Part model, mm, in its own coordinate system. Round coordinates to 2 decimals unless told otherwise and drop trailing zeros. Loops run counter-clockwise (first coordinate to the right, second up) from the corner with the lowest first, then second, coordinate; pieces in that order, holes last.
from build123d import *

# Parameters (mm, degrees)
SKETCH1_W           = 406.4
SKETCH1_H           = 406.4
BOSS_EXTRUDE1_DEPTH = 6.35
CUT_EXTRUDE1_REACH  = 8.35
SKETCH2_R           = 46
SKETCH2_R_2         = 2.15
SKETCH2_R_3         = 2.165


with BuildPart() as part:
    # Sketch1 → Boss-Extrude1 (new body)
    with BuildSketch(Plane(origin=(0, 0, 0), x_dir=(1, 0, 0), z_dir=(0, 1, 0))):
        Rectangle(SKETCH1_W, SKETCH1_H)
    extrude(amount=BOSS_EXTRUDE1_DEPTH)

    # Sketch2 → Cut-Extrude1 (cut, up to next)
    with BuildSketch(Plane(origin=(0, 6.35, 0), x_dir=(1, 0, 0), z_dir=(0, 1, 0)), mode=Mode.PRIVATE) as cut_extrude1_sk1:
        Circle(SKETCH2_R)
    cut_extrude1_tool1 = extrude(cut_extrude1_sk1.sketch, amount=-CUT_EXTRUDE1_REACH, mode=Mode.PRIVATE) & part.part
    add(cut_extrude1_tool1.solids().sort_by_distance((0, 6.35, 0))[0], mode=Mode.SUBTRACT)
    # Sketch2 → Cut-Extrude1 (cut, up to next)
    with BuildSketch(Plane(origin=(0, 6.35, 0), x_dir=(1, 0, 0), z_dir=(0, 1, 0)), mode=Mode.PRIVATE) as cut_extrude1_sk2:
        with Locations((52.5, 52.5)):
            Circle(SKETCH2_R_2)
    cut_extrude1_tool2 = extrude(cut_extrude1_sk2.sketch, amount=-CUT_EXTRUDE1_REACH, mode=Mode.PRIVATE) & part.part
    add(cut_extrude1_tool2.solids().sort_by_distance((52.5, 6.35, -52.5))[0], mode=Mode.SUBTRACT)
    # Sketch2 → Cut-Extrude1 (cut, up to next)
    with BuildSketch(Plane(origin=(0, 6.35, 0), x_dir=(1, 0, 0), z_dir=(0, 1, 0)), mode=Mode.PRIVATE) as cut_extrude1_sk3:
        with Locations((52.5, -52.5)):
            Circle(SKETCH2_R_2)
    cut_extrude1_tool3 = extrude(cut_extrude1_sk3.sketch, amount=-CUT_EXTRUDE1_REACH, mode=Mode.PRIVATE) & part.part
    add(cut_extrude1_tool3.solids().sort_by_distance((52.5, 6.35, 52.5))[0], mode=Mode.SUBTRACT)
    # Sketch2 → Cut-Extrude1 (cut, up to next)
    with BuildSketch(Plane(origin=(0, 6.35, 0), x_dir=(1, 0, 0), z_dir=(0, 1, 0)), mode=Mode.PRIVATE) as cut_extrude1_sk4:
        with Locations((-52.5, -52.5)):
            Circle(SKETCH2_R_2)
    cut_extrude1_tool4 = extrude(cut_extrude1_sk4.sketch, amount=-CUT_EXTRUDE1_REACH, mode=Mode.PRIVATE) & part.part
    add(cut_extrude1_tool4.solids().sort_by_distance((-52.5, 6.35, 52.5))[0], mode=Mode.SUBTRACT)
    # Sketch2 → Cut-Extrude1 (cut, up to next)
    with BuildSketch(Plane(origin=(0, 6.35, 0), x_dir=(1, 0, 0), z_dir=(0, 1, 0)), mode=Mode.PRIVATE) as cut_extrude1_sk5:
        with Locations((-52.5, 52.5)):
            Circle(SKETCH2_R_3)
    cut_extrude1_tool5 = extrude(cut_extrude1_sk5.sketch, amount=-CUT_EXTRUDE1_REACH, mode=Mode.PRIVATE) & part.part
    add(cut_extrude1_tool5.solids().sort_by_distance((-52.5, 6.35, -52.5))[0], mode=Mode.SUBTRACT)


solid = part.part
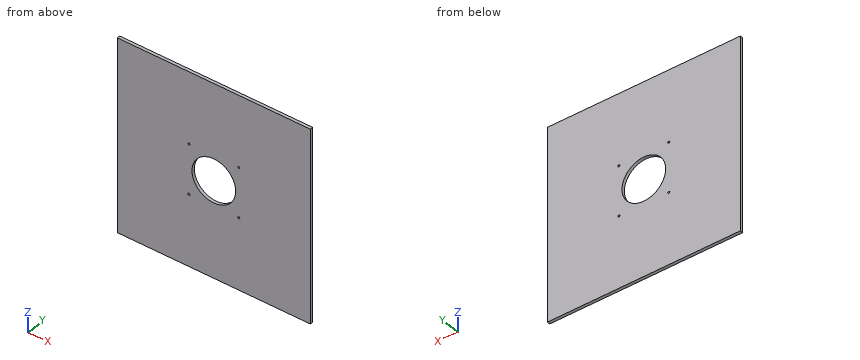
1) Slice it at C-C, the plane y = 2.5. Give the cut face in (x, z) (3 decimals).
Values:
outline: (-203.2, -203.2) - (203.2, -203.2) - (203.2, 203.2) - (-203.2, 203.2) - close; hole circle Ø4.33 at (-52.5, -52.5); hole circle Ø4.3 at (-52.5, 52.5); hole circle Ø92 at (0, 0); hole circle Ø4.3 at (52.5, -52.5); hole circle Ø4.3 at (52.5, 52.5)
2) Slice it at B-B, the plane z = 0. Give the cut face in (x, y), then the cut area to 3 significant figures.
Values:
outline: (-203.2, 0) - (-46, 0) - (-46, 6.35) - (-203.2, 6.35) - close; (46, 0) - (203.2, 0) - (203.2, 6.35) - (46, 6.35) - close
area: 2,000 mm2
3) Slice it at A-A, the plane x = 0. Give the cut face in (y, z).
Values:
outline: (0, -203.2) - (6.35, -203.2) - (6.35, -46) - (0, -46) - close; (0, 46) - (6.35, 46) - (6.35, 203.2) - (0, 203.2) - close
4) Wall check: line 1 along X through (y, z) = (2.25, 52.5); line 2 along X through (y, z) = (4.5, -52.5) (3 decimals). Give the ranges that are in metal, low to high.
Values:
line 1: x = -203.2 to -54.65, -50.35 to 50.35, 54.65 to 203.2
line 2: x = -203.2 to -54.665, -50.335 to 50.35, 54.65 to 203.2
5) Drop a flat-ended pin along its axis: pin 1 Ø2.5 at (x, z) = (52.5, 52.5) entering from -Y. Give the stop position or say it passes through.
Values:
pin 1: passes through
